```python
from build123d import *

# Parameters (mm, degrees)
CUT_EXTRUDE1_DEPTH        = 2.54
CUT_EXTRUDE1_DEPTH_BACK   = 2.54
SKETCH4_W                 = 6.7
SKETCH4_H                 = 0.2
F_2_56_TAPPED_HOLE1_D     = 1.778
F_2_56_TAPPED_HOLE1_DEPTH = 6.604
F_2_56_TAPPED_HOLE1_TIP   = 0.53416509
M2X0_4_TAPPED_HOLE1_D     = 1.6
M2X0_4_TAPPED_HOLE1_DEPTH = 6.096
M2X0_4_TAPPED_HOLE1_TIP   = 0.480688495
SKETCH10_R                = 8.5
BOSS_EXTRUDE2_DEPTH       = 23.622


with BuildPart() as part:
    # Sketch3 → Revolve1 (revolve)
    with BuildSketch(Plane.XY, mode=Mode.PRIVATE) as revolve1_sk:
        Polygon((0, -8.5), (28.5, -8.5), (28.5, -7.25), (30.5, -7.25), (30.5, -8), (32, -8), (32, -3.5), (33.5, -3.5), (33.5, -1.5), (40.888216755, -1.5), (41.661571645, -1.5), (46.2, -1.5), (46.2, 0), (0, 0), align=None)
    revolve(revolve1_sk.sketch.rotate(Axis((0, 0, 0), (1, 0, 0)), 270), axis=Axis((0, 0, 0), (1, 0, 0)))

    # Sketch4 → Cut-Extrude1 (cut, two sides: drawn at the far end of the back side and taken through both)
    with BuildSketch(Plane(origin=(0, 0, 0), x_dir=(1, 0, 0), z_dir=(0, 1, 0)).offset(-CUT_EXTRUDE1_DEPTH_BACK)):
        with Locations((38.55, -1.4)):
            Rectangle(SKETCH4_W, SKETCH4_H)
    extrude(amount=CUT_EXTRUDE1_DEPTH + CUT_EXTRUDE1_DEPTH_BACK, mode=Mode.SUBTRACT)

    # 2-56 Tapped Hole1
    with Locations(Plane(origin=(32, 0, 0), x_dir=(0, 0, -1), z_dir=(1, 0, 0))):
        with Locations((0, 5.46), (0, -5.46)):
            Hole(F_2_56_TAPPED_HOLE1_D / 2, depth=F_2_56_TAPPED_HOLE1_DEPTH)
            with Locations((0, 0, -(F_2_56_TAPPED_HOLE1_DEPTH + F_2_56_TAPPED_HOLE1_TIP / 2))):  # 118° drill point
                Cone(0, F_2_56_TAPPED_HOLE1_D / 2, F_2_56_TAPPED_HOLE1_TIP, mode=Mode.SUBTRACT)

    # M2x0.4 Tapped Hole1
    with Locations(Plane(origin=(32, 0, 0), x_dir=(0, 0, -1), z_dir=(1, 0, 0))):
        with Locations((-5.46, 0), (5.46, 0)):
            Hole(M2X0_4_TAPPED_HOLE1_D / 2, depth=M2X0_4_TAPPED_HOLE1_DEPTH)
            with Locations((0, 0, -(M2X0_4_TAPPED_HOLE1_DEPTH + M2X0_4_TAPPED_HOLE1_TIP / 2))):  # 118° drill point
                Cone(0, M2X0_4_TAPPED_HOLE1_D / 2, M2X0_4_TAPPED_HOLE1_TIP, mode=Mode.SUBTRACT)

    # Sketch10 → Boss-Extrude2 (add)
    with BuildSketch(Plane.ZY):
        Circle(SKETCH10_R)
    extrude(amount=BOSS_EXTRUDE2_DEPTH)


solid = part.part
```
CAD build for the part. Positions are in the model's coordinates, mm. A direction names the side the tool comes from. Coordinates: 2 decimals unless noted, no trailing zeros. Write each loop counter-clockwise with the first axis right and the second up, starting at its lowest first coordinate (ties: lowest second). Pieces come first, ordered by that corner, then holes.
(1) Drill centre lines: probe 1 along Y at (x, z) = (27, 0); probe 2 along X at (y, z) = (-6.75, -4); probe 3 along X at (y, z) = (-4.5, 0.25). Where is each one in solid material? Low to high.
(2) Flat gauge pins, fed straight in: pin 1 (1.8 mm diameter, centred on y = 0, z = -5.46, fed in from +X); pin 2 (8 mm diameter, centred on y = 4.5, z = -2, fed in from +X); pin 3 (1.5 mm diameter, centred on x = 10, y = 3.5, fed in from -Z); pin 4 (1.5 mm diameter, centred on x = 12.5, y = -3, fed in from -Z). Where does each tip first touch, or does it go through?
(3) Cut at A-A, the plane y = -2.25. List the corners of the cut face in (x, z), and give its area (3 significant figures).
(4) 3-axis set-ups, long thin cutter, end or side, ignore diameter. For faces 4 (the face through (29.514, 2.777, 6.697)), 5 (the face through (32, 1.7, 3.4)), 6 (the face through (46.2, 0, 0)): which of +Z, -Z, +X, -X, +Y, -Y reach the whole face in a straight line?
(5) Cut at B-B, the plane x = -3. List the corners of the cut face in (y, z).
(6) Two-plate mould, pull along X, no slides. Class faces 1 (the face through (39, 0, 1.3)), 2 (the face through (28.909, 0.24, 6.223)), 3 (the face through (24.955, -5.611, 0.033)): +X half, -X half, draft (parallel to the pull), parting line (faces both ways), or undercut.
Geometry says:
1. probe 1: y = -8.5 to -6.35, -4.57 to 4.57, 6.35 to 8.5
1. probe 2: x = -23.62 to 28.5, 30.5 to 32
1. probe 3: x = -23.62 to 32
2. pin 1: stops at x = 32
2. pin 2: stops at x = 46.2
2. pin 3: stops at z = -8.04
2. pin 4: stops at z = -8.2
3. outline: (-23.62, -8.2) - (28.5, -8.2) - (28.5, -6.89) - (30.5, -6.89) - (30.5, -7.68) - (32, -7.68) - (32, -2.68) - (33.5, -2.68) - (33.5, 2.68) - (32, 2.68) - (32, 7.68) - (30.5, 7.68) - (30.5, 6.89) - (28.5, 6.89) - (28.5, 8.2) - (-23.62, 8.2) - close
3. area: 913 mm2
4. face 4: none
4. face 5: +X
4. face 6: +Z, -Z, +X, +Y, -Y
5. outline: circle Ø17 at (0, 0)
6. face 1: undercut
6. face 2: draft
6. face 3: +X half
